Geometry check sheet. Reference: the model listing, model coordinates, mm. A direction names the side the tool comes from. Round coordinates to 2 decimals unless told otherwise and drop trailing zeros. Write each loop counter-clockwise with the first axis right and the second up, starting at its lowest first coordinate (ties: lowest second). Pieces come first, ordered by that corner, then holes.
Item 1: Access from +Z, -Z, +X, -X, +Y, -Y to the whole of each face (thin tool, end or side, straight path). Record for faces 1 (the face through (163, -132, -10)), 2 (the face through (-2, -2, 20)), 3 (the face through (146, -265, -22)).
Item 2: Depth check by flat-ended pin: P1, Ø8.5, axis at x = 147.5, z = -22.5, coming from the +Y side; P2, Ø5, axis at x = -70.5, z = -3.5, coming from the -Y side; P3, Ø10, axis at x = -80.5, z = -21, coming from the +Y side; P4, Ø3, axis at x = 43, z = 19, coming from the +Y side. Enter the tip coordinate at first touch or a pass-through.
Item 3: Cross-section at B-B (x = 0). Enter the section's corners in (y, z).
Item 4: Scan lines: probe 1 along X at (y, z) = (-169.5, -22.5); probe 2 along X at (y, z) = (-76, -25); probe 3 along Y at (x, z) = (-1.5, -23.5). Record each from-to range of solid material in increasing order.
Item 5: Draft check along X on faces 4 (the face through (-150, -267, -20)), 5 (the face through (-163, -132, -10)), 6 (the face through (-165, -132, -23)). Enter one of: pulls with the +X half, pulls with the -X half, needs draft (parallel to the pull), parting line crosses it, or undercut.
Item 6: Cross-section at C-C (y = -165.5). State how many separate pieces and enclosed holes the cut face has, then the cut area to 3 significant figures.
Item 7: Cross-section at A-A (y = -54). Enter the section's corners in (x, z).
from build123d import *

# Parameters (mm, degrees)
F1_DEPTH       = 267
F2_W           = 250
F2_H           = 8
F3_DEPTH       = 5
F4_R           = 130
F5_DEPTH       = 12.5
F6_W           = 150
F6_H           = 40
F7_DEPTH       = 2
F8_W           = 40
F8_H           = 10
F9_DEPTH       = 12.5
F10_F1_R       = 5
F10_F2_R       = 5
F10_F3_R       = 4.9999
F10_F4_R       = 4.9999
F10_2_T1_DEPTH = 35
F11_W          = 28.4319519997
F11_H          = 28
F12_DEPTH      = 2
F13_R          = 5
F14_DEPTH      = 5
F17_T1_DEPTH   = 27
F17_T3_DEPTH   = 292
F17_T5_DEPTH   = 60
F20_DEPTH      = 28
F21_T2_ANGLE   = 186.62682558


# Not quite as in the source:
# - a fillet or chamfer that OpenCascade refuses, or shapes differently, is made with other operations: its cross-section is extruded or revolved along the edge and cut away or added
# - a fillet or chamfer is up to 0.001 mm smaller than in the source, because OpenCascade refuses the exact size


with BuildPart() as f1:
    # F0 (on Front) → F1 (new body)
    with BuildSketch(Plane.XZ):
        Polygon((-165, -30), (-163, -30), (-163, -2), (0, -2), (0, 0), (-165, 0), align=None)
    extrude(amount=F1_DEPTH)


with BuildPart() as f3:
    # F2 (on face) → F3 (new body, symmetric)
    with BuildSketch(Plane(origin=(-165, 0, 0), x_dir=(0, -1, 0), z_dir=(-1, 0, 0))):
        with Locations((135, -16)):
            Rectangle(F2_W, F2_H)
    extrude(amount=F3_DEPTH, both=True)

    # F10#2: fillet of radius 5 on 4 edges, made by hand

    # F10_2_s2 → F10_2_t1 (cut)
    with BuildSketch(Plane.YZ.offset(-182.5)):
        with BuildLine():
            ThreePointArc((-15, -12), (-11.4644660941, -13.4644660941), (-10, -17))
            Line((-10, -17), (-10, -12))
            Line((-10, -12), (-15, -12))
        make_face()
        with BuildLine():
            ThreePointArc((-15, -20), (-11.4644660941, -18.5355339059), (-10, -15))
            Line((-10, -15), (-10, -20))
            Line((-10, -20), (-15, -20))
        make_face()
        with BuildLine():
            ThreePointArc((-260, -15), (-258.5355339059, -18.5355339059), (-255, -20))
            Line((-255, -20), (-260, -20))
            Line((-260, -20), (-260, -15))
        make_face()
        with BuildLine():
            ThreePointArc((-255, -12), (-258.5355339059, -13.4644660941), (-260, -17))
            Line((-260, -17), (-260, -12))
            Line((-260, -12), (-255, -12))
        make_face()
    extrude(amount=F10_2_T1_DEPTH, mode=Mode.SUBTRACT)


with BuildPart() as f5:
    # F4 (on face) → F5 (new body, symmetric)
    with BuildSketch(Plane.XY):
        with Locations((0, -267)):
            Circle(F4_R)
    extrude(amount=F5_DEPTH, both=True)


with BuildPart() as f7:
    # F6 (on face) → F7 (new body)
    with BuildSketch(Plane(origin=(0, 0, 0), x_dir=(-1, 0, 0), z_dir=(0, 1, 0))):
        with Locations((75, 20)):
            Rectangle(F6_W, F6_H)
    extrude(amount=-F7_DEPTH)


with BuildPart() as f9:
    # F8 (on face) → F9 (new body, symmetric)
    with BuildSketch(Plane.XZ.offset(2)):
        with Locations((-120, 20)):
            Rectangle(F8_W, F8_H)
    extrude(amount=F9_DEPTH, both=True)

    # F10: fillet of radius 5 on 4 edges, made by hand

    # F10_f1
    f10_f1_edges = [f9.edges().sort_by_distance(p)[0] for p in [
        (-140, -2, 25),
    ]]
    fillet(f10_f1_edges, radius=F10_F1_R)

    # F10_f2
    f10_f2_edges = [f9.edges().sort_by_distance(p)[0] for p in [
        (-100, -2, 25),
    ]]
    fillet(f10_f2_edges, radius=F10_F2_R)

    # F10_f3 (radius 5 in the source; OpenCascade refuses exactly that, so slightly less here)
    f10_f3_edges = [f9.edges().sort_by_distance(p)[0] for p in [
        (-100, -2, 15),
    ]]
    fillet(f10_f3_edges, radius=F10_F3_R)

    # F10_f4 (radius 5 in the source; OpenCascade refuses exactly that, so slightly less here)
    f10_f4_edges = [f9.edges().sort_by_distance(p)[0] for p in [
        (-140, -2, 15),
    ]]
    fillet(f10_f4_edges, radius=F10_F4_R)


with BuildPart() as f12:
    # F11 (on face) → F12 (new body)
    with BuildSketch(Plane.XZ.offset(267)):
        with Locations((-146.2773531675, -16)):
            Rectangle(F11_W, F11_H)
    extrude(amount=-F12_DEPTH)


with BuildPart() as f14:
    # F13 (on face) → F14 (new body, symmetric)
    with BuildSketch(Plane.XZ.offset(267)):
        with Locations((-146.2773531675, -16)):
            Circle(F13_R)
    extrude(amount=F14_DEPTH, both=True)


with BuildPart() as f1_1:
    add(f1.part)

    # F15: union F7, F12
    add(f7.part)
    add(f12.part)

    # F16: cut F9, F3, F5, F14
    add(f9.part, mode=Mode.SUBTRACT)
    add(f3.part, mode=Mode.SUBTRACT)
    add(f5.part, mode=Mode.SUBTRACT)
    add(f14.part, mode=Mode.SUBTRACT)

    # F17: fillet of radius 5 on 3 edges, made by hand

    # F17_s2 → F17_t1 (cut)
    with BuildSketch(Plane.XZ.offset(-12.5)):
        with BuildLine():
            ThreePointArc((-150, 35), (-148.5355339059, 38.5355339059), (-145, 40))
            Line((-145, 40), (-150, 40))
            Line((-150, 40), (-150, 35))
        make_face()
    extrude(amount=F17_T1_DEPTH, mode=Mode.SUBTRACT)

    # F17_s4 → F17_t3 (cut)
    with BuildSketch(Plane.XZ.offset(-12.5)):
        with BuildLine():
            ThreePointArc((-165, -5), (-163.5355339059, -1.4644660941), (-160, 0))
            Line((-160, 0), (-165, 0))
            Line((-165, 0), (-165, -5))
        make_face()
    extrude(amount=F17_T3_DEPTH, mode=Mode.SUBTRACT)

    # F17_s6 → F17_t5 (cut)
    with BuildSketch(Plane.YZ.offset(-177.5)):
        with BuildLine():
            ThreePointArc((-267, -5), (-265.5355339059, -1.4644660941), (-262, 0))
            Line((-262, 0), (-267, 0))
            Line((-267, 0), (-267, -5))
        make_face()
    extrude(amount=F17_T5_DEPTH, mode=Mode.SUBTRACT)

    # F18: F1 across plane


with BuildPart() as f1_2:
    add(f1_1.part)
    add(f1_1.part.mirror(Plane.YZ))

    # F19 (on face) → F20 (join)
    with BuildSketch(Plane(origin=(0, 0, -2), x_dir=(1, 0, 0), z_dir=(0, 0, -1))):
        with BuildLine():
            ThreePointArc((129.9961537893, 266), (0, 137), (-129.9961537893, 266))
            Line((-129.9961537893, 266), (-131.9962120669, 266))
            ThreePointArc((-131.9962120669, 266), (0, 135), (131.9962120669, 266))
            Line((131.9962120669, 266), (129.9961537893, 266))
        make_face()
    extrude(amount=F20_DEPTH)

    # F21: fillet of radius 5 on 1 edges, made by hand

    # F21_s1 → F21_t2 (revolve, cut)
    with BuildSketch(Plane(origin=(15.4061976699, -266.1080656422, 0), x_dir=(0, 0, 1), z_dir=(0.0577977346, -0.9983283137, 0))):
        with BuildLine():
            ThreePointArc((0, 150.4319951252), (-1.4644660941, 146.8964612192), (-5, 145.4319951252))
            Line((-5, 145.4319951252), (0, 145.4319951252))
            Line((0, 145.4319951252), (0, 150.4319951252))
        make_face()
    revolve(axis=Axis((0, -267, 0), (0, 0, -1)), revolution_arc=F21_T2_ANGLE, mode=Mode.SUBTRACT)


solid = f1_2.part
Resolved:
1. face 1: -Z, +Y, -Y
1. face 2: +Z, +X, -X, -Y
1. face 3: -Z, +Y
2. P1: stops at y = -265
2. P2: stops at y = -159.29
2. P3: stops at y = -158.72
2. P4: stops at y = 0
3. outline: (-137, -30) - (-135, -30) - (-135, -2) - (0, -2) - (0, 40) - (-2, 40) - (-2, 0) - (-132, 0) arc R5 ccw to (-137, -5) - close
4. probe 1: x = -165 to -163, -88.98 to -85.99, 85.99 to 88.98, 163 to 165
4. probe 2: x = -165 to -163, 163 to 165
4. probe 3: y = -137.01 to -135.01
5. face 4: needs draft
5. face 5: undercut
5. face 6: pulls with the -X half
6. separate pieces: 4
6. enclosed holes: 0
6. area: 565 mm2
7. outline: (-165, -30) - (-163, -30) - (-163, -20) - (-165, -20) - close; (-165, -12) - (-163, -12) - (-163, -2) - (163, -2) - (163, -12) - (165, -12) - (165, -5) arc R5 ccw to (160, 0) - (-160, 0) arc R5 ccw to (-165, -5) - close; (163, -30) - (165, -30) - (165, -20) - (163, -20) - close
